```python
from build123d import *

# Parameters (mm, degrees)
ENL_V_MAT_EXTRU_1_DEPTH                        = 21.802644063
CONG_1_R                                       = 0.5
FRAISAGE_POUR_VIS_T_TE_FRAIS_E_M21_D           = 2.4
FRAISAGE_POUR_VIS_T_TE_FRAIS_E_M21_CSINK_D     = 4.4
FRAISAGE_POUR_VIS_T_TE_FRAIS_E_M21_CSINK_ANGLE = 90


with BuildPart() as part:
    # Esquisse1 → Révolution1 (revolve)
    with BuildSketch(Plane.XY, mode=Mode.PRIVATE) as r_volution1_sk:
        Polygon((12, 0), (12, 1), (14.5, 1), (14.5, 2.5), (13.5, 3.5), (0, 3.5), (0, 0), align=None)
    revolve(r_volution1_sk.sketch.rotate(Axis((0, -5.347368421, 0), (0, 1, 0)), 90), axis=Axis((0, -5.347368421, 0), (0, 1, 0)))

    # Esquisse2 → Enlèv. mat.-Extru.1 (cut, through all)
    with BuildSketch(Plane(origin=(0, 3.5, 0), x_dir=(1, 0, 0), z_dir=(0, 1, 0))):
        with BuildLine():
            Line((-6, -7.365459931), (-6, 7.365459931))
            ThreePointArc((-6, 7.365459931), (0, 9.5), (6, 7.365459931))
            Line((6, 7.365459931), (6, -7.365459931))
            ThreePointArc((6, -7.365459931), (0, -9.5), (-6, -7.365459931))
        make_face()
    extrude(amount=-ENL_V_MAT_EXTRU_1_DEPTH, mode=Mode.SUBTRACT)

    # Congé1
    cong_1_edges = [part.edges().sort_by_distance(p)[0] for p in [
        (0, 0, 9.5),
        (-6, 0, 0),
        (0, 0, -9.5),
        (6, 0, 0),
        (0, 3.5, 9.5),
        (6, 3.5, 0),
        (0, 3.5, -9.5),
        (-6, 3.5, 0),
        (0, 2.5, 14.5),
        (0, 3.5, 13.5),
    ]]
    fillet(cong_1_edges, radius=CONG_1_R)

    # Fraisage pour vis à tête fraisée M21 (through all)
    with Locations(Plane(origin=(-9, 3.5, 0), x_dir=(0, 0, 1), z_dir=(0, 1, 0))):
        with Locations((0, 0), (0, 18)):
            CounterSinkHole(FRAISAGE_POUR_VIS_T_TE_FRAIS_E_M21_D / 2, FRAISAGE_POUR_VIS_T_TE_FRAIS_E_M21_CSINK_D / 2, counter_sink_angle=FRAISAGE_POUR_VIS_T_TE_FRAIS_E_M21_CSINK_ANGLE)


solid = part.part
```
Can you work these out from the model? Positions are in its coordinate system, mm. A direction names the side the tool comes from. Give positions to 0.01 mm unless a question says otherwise; leave off trailing zeros. Order: outer loops, then holes, each group sorted by start corner. A loop starts at its lowest first (then second) coordinate and runs counter-clockwise, first axis right, second up. Notation, with made-up numbers: M 5.25,76 L 23.25,76 A18 ccw 23.25,86 Z; hole C -19,10.5 d7. An arc over 180 degrees is marked long. Write item = value, one per line. Start each with the question number.
Q1. We'd pull the mould along X, two halves only. Please class faces 4 (the cylindrical face through (-3.604, 0.507, -11.446)), 5 (the cylindrical face through (-0.1, 1.8, -9.5)), 6 (the flat face through (7, 0, 1)): pulls with the +X half, pulls with the -X half, needs draft (parallel to the pull), parting line crosses it, or undercut.
Q2. For faces 1 (the flat face through (9, 3.5, -3)), 2 (the cylindrical face through (0.1, 1.8, 9.5)), 3 (the flat face through (-12, 1, 2)), which set-ups out of +Z, -Z, +X, -X, +Y, -Y let a thin tool reach every point of the face, with its end or its side?
Q3. Suppose I cut it at B-B (z = 0). Count the separate pieces of the cut face and the enclosed holes in it, plus the area to 3 significant figures.
Q4. I need wall thicknesses on probe 1 along X at (y, z) = (0.85, 0); probe 2 along X at (y, z) = (1.7, 0); probe 3 along Z at (x, y) = (9, 1.4). Which ranges of each line are inside material? Lowest first, please. Write a range as [from, to].
Q5. Will these pins go through, and if not, where does the flat tip stop? pin 1 Ø2 at (x, y) = (-3.5, 3) entering from +Z; pin 2 Ø2 at (x, y) = (-4.5, 2.5) entering from +Z; pin 3 Ø0.7 at (y, z) = (1.5, -3.5) entering from +X.
Q6. Suppose I cut it at A-A (y = 1.7). Write out the boundary of the cut face in (x, z), plus the area to 3 significant figures.
Check result:
q1.face_4 = parting line crosses it
q1.face_5 = undercut
q1.face_6 = needs draft
q2.face_1 = +Z, -Z, +X, -X, +Y
q2.face_2 = +Y, -Y
q2.face_3 = -Y
q3.separate_pieces = 4
q3.enclosed_holes = 0
q3.area = 34.5 mm2
q4.probe_1 = [-12, -10.2], [-7.8, -6], [6, 7.8], [10.2, 12]
q4.probe_2 = [-14.5, -10.2], [-7.8, -6], [6, 7.8], [10.2, 14.5]
q4.probe_3 = [-11.37, -1.2], [1.2, 11.37]
q5.pin_1 = 14.24
q5.pin_2 = 14.07
q5.pin_3 = 14.15
q6.outline = C 0,0 d29; hole C -9,0 d2.4; hole M -6,-7.37 A9.5 ccw 6,-7.37 L 6,7.37 A9.5 ccw -6,7.37 Z; hole C 9,0 d2.4
q6.area = 440 mm2
